Autodesk Inventor part; units mm, degrees
ref_plane "YZ Plane" through (0, 0, 0) normal (1, 0, 0) x (0, 1, 0)
ref_plane "XZ Plane" through (0, 0, 0) normal (0, 1, 0) x (-1, 0, 0)
ref_plane "XY Plane" through (0, 0, 0) normal (0, 0, 1) x (1, 0, 0)
sketch "Sketch1" plane through (0, 0, 0) normal (0, 1, 0) x (-1, 0, 0)
  circle A0 centre (0, 0) radius 12.02
  circle A1 centre (0, 0) radius 4
  dimension "d0" = 24.04
  dimension "d1" = 8
extrude "Extrusion1" add sketch "Sketch1" along normal blind 9
sketch "Sketch2" plane through (0, 9, 0) normal (0, 1, 0) x (1, 0, 0)
  circle A0 centre (0, 0) radius 4
  circle A1 centre (0, 0) radius 9
  circle A2 centre (0, 0) radius 4
  dimension "d4" = 18
extrude "Extrusion2" add sketch "Sketch2" along normal blind 9
sketch "Sketch3" plane through (0, 18, 0) normal (0, 1, 0) x (1, 0, 0)
  circle A0 centre (0, 0) radius 6.5
  dimension "d7" = 13
extrude "Extrusion3" cut sketch "Sketch3" against normal blind 10
fillet "Fillet1" radius 0.5 5 edges at (4, 0, 0) (12.02, 0, 0) (12.02, 9, 0) (-9, 9, 0) (-9, 18, 0)
properties part number "Z-Zahnrad"
Work out the finished part from the listing and answer in its coordinate system (mm). A direction names the side the tool comes from. Give positions to 0.01 mm unless a question says otherwise; leave off trailing zeros. Loops run counter-clockwise (first coordinate to the right, second up) from the corner with the lowest first, then second, coordinate; pieces in that order, holes last. Notation, with made-up numbers: (8.25, 62) - (33.25, 62) arc R17 ccw to (33.25, 89) - close; hole circle Ø4 at (3, 29). An arc over 180 degrees is marked (long way). Use CSV: the item, a comma, the result in double quotes. Start each with the question number.
(1) A tool of negligible diameter and unlimited length cuts with its end or side. For faces 4 (the face through (-11.465, 4.444, -3.61)), 5 (the face through (3, 8, -3)), from which of +Z, -Z, +X, -X, +Y, -Y can it reach the whole face along a straight path? Write none if from no direction.
(2) Find the intervals of material crossed by L1, parallel to Z at x = 0, y = 16; L2, parallel to Z at x = 0, y = 3.75; L3, parallel to Y at x = -1.75, z = 4.25, in increasing order.
(3) Find section D-D, the plane y = 13.5. Determine the outline of the cut face in (x, z).
(4) Find section B-B, the plane x = 0. Determine the outline of the cut face in (y, z), plus the area to 3 significant figures.
(5) Find section C-C, the plane y = 2. Determine the outline of the cut face in (x, z), plus the area to 3 significant figures.
(6) Find section A-A, the plane z = 0. Determine the outline of the cut face in (x, y), plus the area to 3 significant figures.
(7) Determine the mould class of faces 1 (the face through (0.867, 4.198, 3.905)), 2 (the face through (4, 9, 9)), 3 (the face through (-1.172, 13.444, 8.923)) for opening direction X: released by +X, released by -X, zero draft, split by the parting line, or undercut.
(8) Each of these flat-tipped pins is pushed along its axis until it touches: pin 1 (8 mm diameter, centred on x = 3, y = 12, fed in from -Z); pin 2 (6 mm diameter, centred on x = -5, y = 7, fed in from +Z); pin 3 (10.5 mm diameter, centred on x = 0, z = 0, fed in from +Y). Where does it stop, or does it pass through?
Results found:
1,face 4,"+Y, -Y"
1,face 5,"+Y"
2,L1,"-9 to -6.5, 6.5 to 9"
2,L2,"-12.02 to -4, 4 to 12.02"
2,L3,"0 to 8"
3,outline,"circle Ø18 at (0, 0); hole circle Ø13 at (0, 0)"
4,outline,"(0, -11.52) arc R0.5 ccw to (0.5, -12.02) - (8.5, -12.02) arc R0.5 ccw to (9, -11.52) - (9, -9.5) arc R0.5 cw to (9.5, -9) - (17.5, -9) arc R0.5 ccw to (18, -8.5) - (18, -6.5) - (8, -6.5) - (8, -4) - (0.5, -4) arc R0.5 ccw to (0, -4.5) - close; (0, 4.5) arc R0.5 ccw to (0.5, 4) - (8, 4) - (8, 6.5) - (18, 6.5) - (18, 8.5) arc R0.5 ccw to (17.5, 9) - (9.5, 9) arc R0.5 cw to (9, 9.5) - (9, 11.52) arc R0.5 ccw to (8.5, 12.02) - (0.5, 12.02) arc R0.5 ccw to (0, 11.52) - close"
4,area,"184 mm^2"
5,outline,"circle Ø24.04 at (0, 0); hole circle Ø8 at (0, 0)"
5,area,"404 mm^2"
6,outline,"(-12.02, 0.5) arc R0.5 ccw to (-11.52, 0) - (-4.5, 0) arc R0.5 ccw to (-4, 0.5) - (-4, 8) - (-6.5, 8) - (-6.5, 18) - (-8.5, 18) arc R0.5 ccw to (-9, 17.5) - (-9, 9.5) arc R0.5 cw to (-9.5, 9) - (-11.52, 9) arc R0.5 ccw to (-12.02, 8.5) - close; (4, 0.5) arc R0.5 ccw to (4.5, 0) - (11.52, 0) arc R0.5 ccw to (12.02, 0.5) - (12.02, 8.5) arc R0.5 ccw to (11.52, 9) - (9.5, 9) arc R0.5 cw to (9, 9.5) - (9, 17.5) arc R0.5 ccw to (8.5, 18) - (6.5, 18) - (6.5, 8) - (4, 8) - close"
6,area,"184 mm^2"
7,face 1,"undercut"
7,face 2,"zero draft"
7,face 3,"split by the parting line"
8,pin 1,"z = -11.98"
8,pin 2,"z = 11.85"
8,pin 3,"y = 8"
